Check sheet for the modelled part. Datum: model origin and axes. Units: mm. Give positions to 0.01 mm unless a question says otherwise; leave off trailing zeros. Order: outer loops, then holes, each group sorted by start corner. A loop starts at its lowest first (then second) coordinate and runs counter-clockwise, first axis right, second up.
```python
from build123d import *

# Parameters (mm, degrees)
F0_R     = 31.5
F1_DEPTH = 27
F2_SIZE2 = 5.7735026919
F2_SIZE  = 10
F3_R     = 2


with BuildPart() as f1:
    # F0 (on Top) → F1 (new body)
    with BuildSketch(Plane.XY):
        Circle(F0_R)
    extrude(amount=F1_DEPTH)

    # F2
    f2_edges = [f1.edges().sort_by_distance(p)[0] for p in [
        (-31.5, 0, 27),
    ]]
    f2_side = f1.faces().sort_by_distance((0, 0, 27))[0]
    chamfer(f2_edges, length=F2_SIZE, length2=F2_SIZE2, reference=f2_side)

    # F3
    f3_edges = [f1.edges().sort_by_distance(p)[0] for p in [
        (-31.5, 0, 0),
    ]]
    fillet(f3_edges, radius=F3_R)


solid = f1.part
```
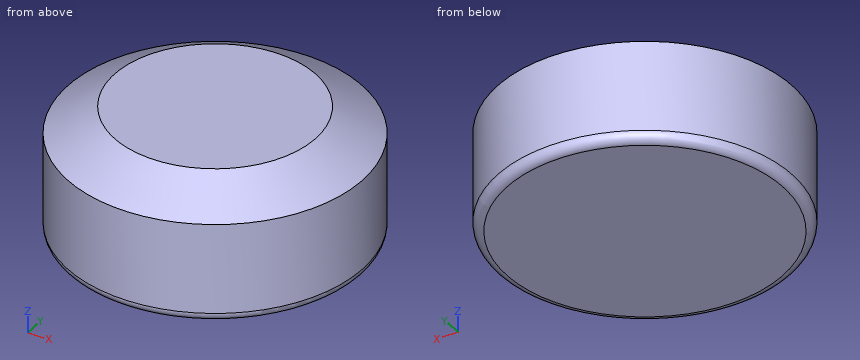
(1) Sectioned sample at C-C (z = 3.75). Enter the section's corners in (x, y).
(2) Sectioned sample at A-A (y = 0). Enter the section's corners in (x, z), plus the area to 3 significant figures.
(3) Thickness scan on L1, parallel to Y at x = 6, z = 13.75; L2, parallel to X at y = 13.5, z = 17.25; L3, parallel to Y at x = -13, z = 12.5. Record the ranges inside material, lowest first.
(4) Go/stop test with flat-tipped pins: P1, Ø8, axis at x = 6.5, z = 21.5, coming from the -Y side; P2, Ø1, axis at y = -17.5, z = 15.5, coming from the -X side; P3, Ø10, axis at y = -7, z = 15.5, coming from the -X side. Record where each tip stops, or that it passes through.
Values follow:
1. outline: circle Ø63 at (0, 0)
2. outline: (-31.5, 2) arc R2 ccw to (-29.5, 0) - (29.5, 0) arc R2 ccw to (31.5, 2) - (31.5, 21.23) - (21.5, 27) - (-21.5, 27) - (-31.5, 21.23) - close
2. area: 1,640 mm2
3. L1: y = -30.92 to 30.92
3. L2: x = -28.46 to 28.46
3. L3: y = -28.69 to 28.69
4. P1: stops at y = -31.4
4. P2: stops at x = -26.52
4. P3: stops at x = -31.44
